Work out the finished part from the listing and answer in its coordinate system (mm). Face numbers are marked on the shaded views. A direction names the side the tool comes from. Give positions to 0.01 mm unless a question says otherwise; leave off trailing zeros. Order: outer loops, then holes, each group sorted by start corner. A loop starts at its lowest first (then second) coordinate and runs counter-clockwise, first axis right, second up. Notation, with made-up numbers: (67.25, -26) - (117.25, -26) arc R30 ccw to (117.25, 9) - close; hole circle Ø3 at (-14.75, 9.5). An arc over 180 degrees is marked (long way). Put each result on its own line as item: value.
```python
from build123d import *

# Parameters (mm, degrees)
SKETCH2_R           = 2.1
BOSS_EXTRUDE1_DEPTH = 26
SKETCH3_W           = 7.4
SKETCH3_H           = 18
SKETCH3_W_2         = 7.8
SKETCH3_W_3         = 7.481047655
CUT_EXTRUDE1_DEPTH  = 17
SKETCH4_W           = 26
SKETCH4_H           = 16
BOSS_EXTRUDE2_DEPTH = 25
SKETCH5_W           = 19
SKETCH5_H           = 6.5
CUT_EXTRUDE2_DEPTH  = 25
FILLET2_R           = 3
SKETCH6_R           = 1.5
CUT_EXTRUDE3_DEPTH  = 12.5
FILLET3_R           = 0.5
FILLET4_R           = 3
CUT_EXTRUDE4_DEPTH  = 3


with BuildPart() as part:
    # Sketch2 → Boss-Extrude1 (new body, symmetric)
    with BuildSketch(Plane(origin=(0, 0, 0), x_dir=(0, 0, -1), z_dir=(1, 0, 0))):
        with BuildLine():
            Line((-8, 0), (-8, 20))
            Line((-8, 20), (8, 20))
            Line((8, 20), (8, 0))
            ThreePointArc((8, 0), (0, -8), (-8, 0))
        make_face()
        Circle(SKETCH2_R, mode=Mode.SUBTRACT)
    extrude(amount=BOSS_EXTRUDE1_DEPTH, both=True)

    # Sketch3 → Cut-Extrude1 (cut, through all)
    with BuildSketch(Plane.XY.offset(8)):
        with Locations((-22.3, 0)):
            Rectangle(SKETCH3_W, SKETCH3_H)
        with Locations((-7.5, 0)):
            Rectangle(SKETCH3_W_2, SKETCH3_H)
        with Locations((7.5, 0)):
            Rectangle(SKETCH3_W_2, SKETCH3_H)
        with Locations((22.259476173, 0)):
            Rectangle(SKETCH3_W_3, SKETCH3_H)
    extrude(amount=-CUT_EXTRUDE1_DEPTH, mode=Mode.SUBTRACT)

    # Sketch4 → Boss-Extrude2 (add)
    with BuildSketch(Plane(origin=(0, 20, 0), x_dir=(1, 0, 0), z_dir=(0, 1, 0))):
        Rectangle(SKETCH4_W, SKETCH4_H)
    extrude(amount=BOSS_EXTRUDE2_DEPTH)

    # Sketch5 → Cut-Extrude2 (cut)
    with BuildSketch(Plane(origin=(0, 45, 0), x_dir=(1, 0, 0), z_dir=(0, 1, 0))):
        Rectangle(SKETCH5_W, SKETCH5_H)
    extrude(amount=-CUT_EXTRUDE2_DEPTH, mode=Mode.SUBTRACT)

    # Fillet2
    fillet2_edges = [part.edges().sort_by_distance(p)[0] for p in [
        (26, 20, 0),
        (-26, 20, 0),
    ]]
    fillet(fillet2_edges, radius=FILLET2_R)

    # Sketch6 → Cut-Extrude3 (cut, symmetric)
    with BuildSketch(Plane.XY):
        with Locations((0, 37.5)):
            Circle(SKETCH6_R)
        with Locations((0, 27.5)):
            Circle(SKETCH6_R)
    extrude(amount=CUT_EXTRUDE3_DEPTH, both=True, mode=Mode.SUBTRACT)

    # Fillet3
    fillet3_edges = [part.edges().sort_by_distance(p)[0] for p in [
        (-13, 45, 0),
        (0, 45, 8),
        (13, 45, 0),
        (0, 45, -8),
    ]]
    fillet(fillet3_edges, radius=FILLET3_R)

    # Fillet4
    fillet4_edges = [part.edges().sort_by_distance(p)[0] for p in [
        (-13, 20, 0),
        (13, 20, 0),
    ]]
    fillet(fillet4_edges, radius=FILLET4_R)

    # Sketch7 → Cut-Extrude4 (cut)
    with BuildSketch(Plane.XY.offset(8)):
        Polygon((3, 35.767949192), (3, 39.232050808), (0, 40.964101615), (-3, 39.232050808), (-3, 35.767949192), (0, 34.035898385), align=None)
        Polygon((3, 25.767949192), (3, 29.232050808), (0, 30.964101615), (-3, 29.232050808), (-3, 25.767949192), (0, 24.035898385), align=None)
    extrude(amount=-CUT_EXTRUDE4_DEPTH, mode=Mode.SUBTRACT)


solid = part.part
```
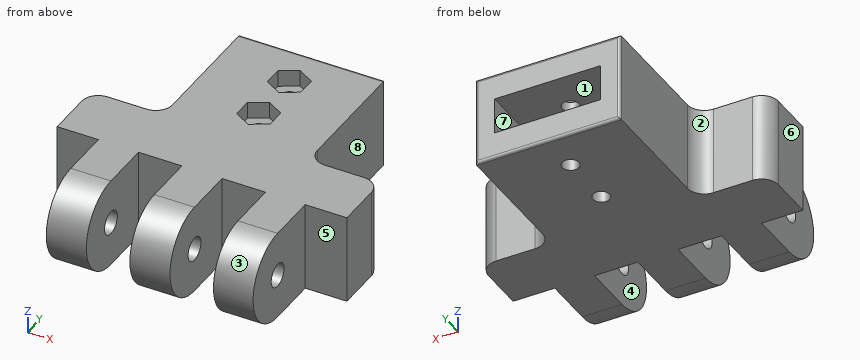
(1) Given pin 1 (1 mm diameter, centred on x = -18.5, z = -0.5, fed in from +Y); pin 2 (3 mm diameter, centred on x = -0.5, y = 27.5, fed in from +Z); pin 3 (3.5 mm diameter, centred on y = 27, z = 6.5, fed in from -X), each flat-ended and moving along its own axis, determine where each tip first touches the part or whether it passes through.
Geometry check:
pin 1: stops at y = 20
pin 2: stops at z = 5
pin 3: stops at x = -13
(2) Straight lines are drawn through the part: line 1 (X direction, y = 3.5, z = -1.75); line 2 (Z direction, x = -2, y = 24.5); line 3 (Y direction, x = 2.25, z = 0). For each, find the intervals that lie inside material, in ascending order.
Geometry check:
line 1: x = -18.6 to -11.4, -3.6 to 3.6, 11.4 to 18.52
line 2: z = -8 to -3.25, 3.25 to 8
line 3: y = -8 to -2.1, 2.1 to 20
(3) A tool of negligible diameter and unlimited length cuts with its end or side. For the marked faces 4, 5, 6, 7 and 8, from which of +Z, -Z, +X, -X, +Y, -Y can it reach the whole face along a straight path? Write none if from no direction.
Geometry check:
face 4: +Z, -Z, -Y
face 5: +Z, -Z, +X, -Y
face 6: +Z, -Z, -X, +Y, -Y
face 7: +Y
face 8: +Z, -Z, +X, +Y
(4) Section A-A, the plane y = 37.5 is taken. Write down the section's boundary in (x, z), then the cut area to 3 significant figures.
Geometry check:
outline: (-13, -8) - (-1.5, -8) - (-1.5, -3.25) - (-9.5, -3.25) - (-9.5, 3.25) - (-1.5, 3.25) - (-1.5, 5) - (-3, 5) - (-3, 8) - (-13, 8) - close; (1.5, -8) - (13, -8) - (13, 8) - (3, 8) - (3, 5) - (1.5, 5) - (1.5, 3.25) - (9.5, 3.25) - (9.5, -3.25) - (1.5, -3.25) - close
area: 255 mm²
(5) Determine the mould class of the marked faces 1, 2 and 3 for opening direction X: pulls with the +X half, pulls with the -X half, needs draft (parallel to the pull), parting line crosses it, or undercut.
Geometry check:
face 1: undercut
face 2: pulls with the -X half
face 3: needs draft
(6) Section B-B, the plane z = 0 is taken. Count the separate pieces of the cut face and the enclosed holes in it, then the cut area to 3 significant figures.
Geometry check:
separate pieces: 4
enclosed holes: 0
area: 1,020 mm²
